from build123d import *

# Parameters (mm, degrees)
ENL_V_MAT_EXTRU_1_DEPTH = 16.5


with BuildPart() as part:
    # Sketch1 → Revolve1 (revolve)
    with BuildSketch(Plane.XY, mode=Mode.PRIVATE) as revolve1_sk:
        Polygon((4, 19.2), (17.5, 19.2), (17.5, 16.2), (15, 16.2), (15, 0), (9, 0), (5, -4), (4, -4), align=None)
    revolve(revolve1_sk.sketch.rotate(Axis((0, 12.709342281, 0), (0, -1, 0)), 90), axis=Axis((0, 12.709342281, 0), (0, -1, 0)))

    # Esquisse1 → Enlèv. mat.-Extru.1 (cut)
    with BuildSketch(Plane(origin=(0, 19.2, 0), x_dir=(1, 0, 0), z_dir=(0, 1, 0))):
        with BuildLine():
            Line((-1.5, 5.4), (-1.5, 3.708099244))
            ThreePointArc((-1.5, 3.708099244), (0, 4), (1.5, 3.708099244))
            Line((1.5, 3.708099244), (1.5, 5.4))
            Line((1.5, 5.4), (-1.5, 5.4))
        make_face()
    extrude(amount=-ENL_V_MAT_EXTRU_1_DEPTH, mode=Mode.SUBTRACT)


solid = part.part
Check sheet for the modelled part. Datum: model origin and axes. Units: mm. A direction names the side the tool comes from. Round coordinates to 2 decimals unless told otherwise and drop trailing zeros. Order: outer loops, then holes, each group sorted by start corner. A loop starts at its lowest first (then second) coordinate and runs counter-clockwise, first axis right, second up.
(1) Access from +Z, -Z, +X, -X, +Y, -Y to the whole of each face (thin tool, end or side, straight path). Record for faces 1 (the cylindrical face through (17.084, 17.679, -3.794)), 2 (the cylindrical face through (-12.65, 7.99, 8.06)), 3 (the flat face through (0, 11, -5.4)).
(2) Scan lines: probe 1 along X at (y, z) = (12.5, 0); probe 2 along Y at (x, z) = (-6.5, 15.5); probe 3 along Y at (x, z) = (10, -8.5). Record each from-to range of solid material in increasing order.
(3) Cross-section at B-B, the plane z = 0. Enter the section's corners in (x, y), and give its area (3 significant figures).
(4) Draft check along X on faces 4 (the conical face through (4.608, -3.806, 2.397)), 5 (the flat face through (-8, 16.2, 13)), 6 (the flat face through (-1.5, 11, -5)). Enter one of: pulls with the +X half, pulls with the -X half, needs draft (parallel to the pull), parting line crosses it, or undercut.
(5) Cross-section at C-C, the plane y = 5.5. Enter the section's corners in (x, z), and give its area (3 significant figures).
(6) Cross-section at D-D, the plane z = 14.5. Enter the section's corners in (x, y).
(7) Cross-section at A-A, the plane x = 0. Enter the section's corners in (y, z).
(8) Go/stop test with flat-tipped pins: P1, Ø0.5, axis at y = 11.5, z = -4.5, coming from the -X side; P2, Ø4, axis at x = -12.5, z = 8, coming from the -Y side; P3, Ø1.4, axis at y = 10, z = -4.5, coming from the +X side. Record where each tip stops, or that it passes through.
Check sheet entries:
1. face 1: +Y, -Y
1. face 2: -Y
1. face 3: +Y
2. probe 1: x = -15 to -4, 4 to 15
2. probe 2: y = 16.2 to 19.2
2. probe 3: y = 0 to 19.2
3. outline: (-17.5, 16.2) - (-15, 16.2) - (-15, 0) - (-9, 0) - (-5, -4) - (-4, -4) - (-4, 19.2) - (-17.5, 19.2) - close; (4, -4) - (5, -4) - (9, 0) - (15, 0) - (15, 16.2) - (17.5, 16.2) - (17.5, 19.2) - (4, 19.2) - close
3. area: 461 mm2
4. face 4: parting line crosses it
4. face 5: needs draft
4. face 6: undercut
5. outline: circle Ø30 at (0, 0); hole (-1.5, -5.4) - (1.5, -5.4) - (1.5, -3.71) arc R4 ccw (long way) to (-1.5, -3.71) - close
5. area: 652 mm2
6. outline: (-9.8, 16.2) - (-3.84, 16.2) - (-3.84, 0) - (3.84, 0) - (3.84, 16.2) - (9.8, 16.2) - (9.8, 19.2) - (-9.8, 19.2) - close
7. outline: (-4, -5) - (0, -9) - (0, -15) - (16.2, -15) - (16.2, -17.5) - (19.2, -17.5) - (19.2, -5.4) - (2.7, -5.4) - (2.7, -4) - (-4, -4) - close; (-4, 4) - (19.2, 4) - (19.2, 17.5) - (16.2, 17.5) - (16.2, 15) - (0, 15) - (0, 9) - (-4, 5) - close
8. P1: stops at x = -14.39
8. P2: stops at y = 0
8. P3: stops at x = 14.51
